Here's how the part is built. I have some questions about the finished solid (model axes, mm). A direction names the side the tool comes from. Give positions to 0.01 mm unless a question says otherwise; leave off trailing zeros. Write each loop counter-clockwise with the first axis right and the second up, starting at its lowest first coordinate (ties: lowest second). Pieces come first, ordered by that corner, then holes. Notation, with made-up numbers: (54, 81.5) - (75, 81.5) arc R19 ccw to (75, 86.5) - close; hole circle Ø9 at (-34.75, 80.5). An arc over 180 degrees is marked (long way). Use a Markdown table: item, result.
```python
from build123d import *

# Parameters (mm, degrees)
F1_DEPTH = 5
F2_R     = 12.7


with BuildPart() as f1:
    # F0 (on Front) → F1 (new body)
    with BuildSketch(Plane.XZ):
        with BuildLine():
            Line((0, -2.056562), (0, 0))
            Line((0, 0), (-40.835929, 30.216998))
            ThreePointArc((-40.835929, 30.216998), (-44.716703, 20.056998), (-40.835929, 9.896998))
            Line((-40.835929, 9.896998), (0, -20.32))
            Line((0, -20.32), (0, -15.264398))
            ThreePointArc((0, -15.264398), (-6.636931, -8.66048), (0, -2.056562))
        make_face()
        with BuildLine():
            Line((40.835929, 30.216998), (0, 0))
            Line((0, 0), (0, -2.056562))
            ThreePointArc((0, -2.056562), (4.64843, -4.002405), (6.571069, -8.66048))
            ThreePointArc((6.571069, -8.66048), (4.64843, -13.318556), (0, -15.264398))
            Line((0, -15.264398), (0, -20.32))
            Line((0, -20.32), (40.835929, 9.896998))
            ThreePointArc((40.835929, 9.896998), (44.716703, 20.056998), (40.835929, 30.216998))
        make_face()
    extrude(amount=F1_DEPTH)

    # F2
    f2_edges = [f1.edges().sort_by_distance(p)[0] for p in [
        (0, -2.5, -20.32),
        (0, -2.5, 0),
    ]]
    fillet(f2_edges, radius=F2_R)


solid = f1.part
```
Item 1: If we section it at D-D, the plane x = -17.5: Write out the boundary of the cut face in (y, z), plus the area to 3 significant figures.
Values:
| item | result |
|---|---|
| outline | (-5, -7.37) - (0, -7.37) - (0, 12.95) - (-5, 12.95) - close |
| area | 102 mm2 |
Item 2: If we section it at C-C, the plane x = 1: Write out the boundary of the cut face in (y, z), plus the area to 3 significant figures.
Values:
| item | result |
|---|---|
| outline | (-5, -17.18) - (0, -17.18) - (0, -15.18) - (-5, -15.18) - close; (-5, -2.14) - (0, -2.14) - (0, 3.14) - (-5, 3.14) - close |
| area | 36.4 mm2 |
Item 3: If we section it at B-B, the plane y = -3.9: Write out the boundary of the cut face in (x, z).
Values:
| item | result |
|---|---|
| outline | (-40.84, 9.9) - (-7.55, -14.73) arc R12.7 ccw to (7.55, -14.73) - (40.84, 9.9) arc R15.24 ccw to (40.84, 30.22) - (7.55, 5.59) arc R12.7 cw to (-7.55, 5.59) - (-40.84, 30.22) arc R15.24 ccw to start; hole (0, -2.06) arc R6.6 ccw (long way) to (6.57, -8.66) arc R6.6 ccw to start |
Item 4: If we section it at A-A, the plane z = 4.5: Write out the boundary of the cut face in (x, y).
Values:
| item | result |
|---|---|
| outline | (-33.54, -5) - (-5.8, -5) - (-5.8, 0) - (-33.54, 0) - close; (5.8, -5) - (33.54, -5) - (33.54, 0) - (5.8, 0) - close |
Item 5: Thinking about a two-plate mould opening in X: for faces 3 (the flat face through (-1, 0, 2)), 4 (the cylindrical face through (-0.11, -2.54, -17.22)), 5 (the flat face through (-24.428, -2.465, -2.244)), 6 (the flat face through (24.428, -2.465, 18.076)), which applies, +X half, -X half, draft (parallel to the pull), parting line (faces both ways), or undercut?
Values:
| item | result |
|---|---|
| face 3 | draft |
| face 4 | parting line |
| face 5 | -X half |
| face 6 | undercut |
Item 6: Will these pins go through, and if not, where does the flat tip stop? pin 1 Ø1 at (x, y) = (-33.5, -3) entering from +Z; pin 2 Ø2 at (x, z) = (18.5, 16) entering from +Y; pin 3 Ø3 at (y, z) = (-1.5, -10.5) entering from -X; pin 4 Ø3 at (x, y) = (26.5, -3) entering from +Z.
Values:
| item | result |
|---|---|
| pin 1 | stops at z = 25.16 |
| pin 2 | passes through |
| pin 3 | stops at x = -15.3 |
| pin 4 | stops at z = 20.72 |
Item 7: I need wall thicknesses on line 1 along Z through (x, y) = (-3, -3.45); line 2 along X through (y, z) = (-4.05, 23); line 3 along X through (y, z) = (-4.25, 15). Which ranges of each line are inside material? Lowest first, please. Write a range as [from, to].
Values:
| item | result |
|---|---|
| line 1 | z = [-16.86, -14.56], [-2.76, 3.46] |
| line 2 | x = [-44.43, -31.08], [31.08, 44.43] |
| line 3 | x = [-43.85, -20.27], [20.27, 43.85] |
Item 8: For faces 1 (the flat face through (-23.96, -2.46, 17.73)), 2 (the cylindrical face through (-44.716, -2.465, 20.213)), which set-ups out of +Z, -Z, +X, -X, +Y, -Y let a thin tool reach every point of the face, with its end or its side?
Values:
| item | result |
|---|---|
| face 1 | +Z, +Y, -Y |
| face 2 | -X, +Y, -Y |
